Design review of the part shown in the three views and the two pictorial views. Dimensions are in mm from the part's minimum x, y and z. A direction names the side the tool comes from. Round coordinates to 2 decimals unless told otherwise and drop trailing zeros. Order: outer loops, then holes, each group sorted by start corner. A loop starts at its lowest first (then second) coordinate and runs counter-clockwise, first axis right, second up.
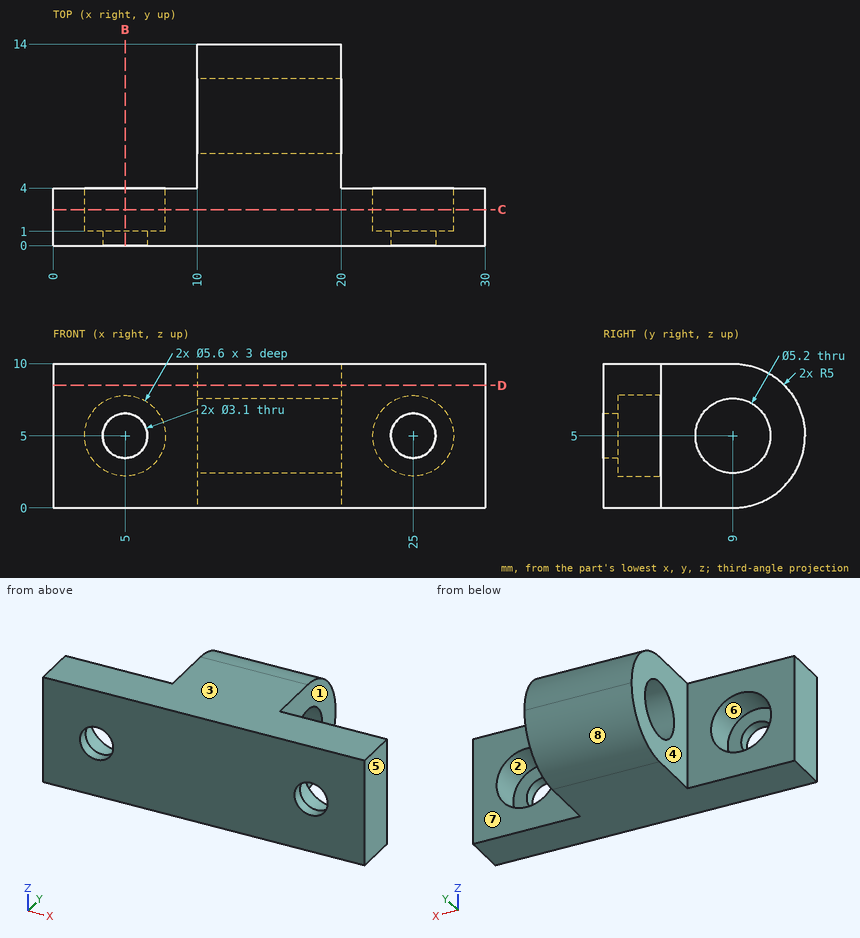
1) The part is to be moulded in two halves that separate along X. For the marked faces 1, 2 and 3, say which applies: released by +X, released by -X, zero draft, split by the parting line, or undercut.
Results:
face 1: released by +X
face 2: undercut
face 3: zero draft
2) To check wall thickness, follow line 1 along X through (y, z) = (2.75, 5); line 2 along Z through (x, y) = (5, 0.6); line 3 along Y through (x, z) = (14, 5). State the ranges of each line that lie inside material, in increasing order.
Results:
line 1: x = 0 to 2.2, 7.8 to 22.2, 27.8 to 30
line 2: z = 0 to 3.45, 6.55 to 10
line 3: y = 0 to 6.4, 11.6 to 14
3) Take a section at D-D on z = 8.5. Give the boundary of the cut face in (x, y), plus the area to 3 significant figures.
Results:
outline: (0, 0) - (30, 0) - (30, 4) - (20, 4) - (20, 12.57) - (10, 12.57) - (10, 4) - (0, 4) - close
area: 206 mm2
4) For the marked faces 4, 5, 6, 7 and 8, list the 3-axis set-ups (+Z, -Z, +X, -X, +Y, -Y) from which the entire face can be reached by the end or side of a thin tool; tool diameter is ignored.
Results:
face 4: +Z, -Z, -X, +Y
face 5: +Z, -Z, +X, +Y, -Y
face 6: +Y
face 7: +Z, -Z, +X, +Y
face 8: -Z, +X, -X, +Y
5) Take a section at C-C on y = 2.5. Give the boundary of the cut face in (x, z).
Results:
outline: (0, 0) - (30, 0) - (30, 10) - (0, 10) - close; hole circle Ø5.6 at (5, 5); hole circle Ø5.6 at (25, 5)
6) Take a section at B-B on x = 5. Give the boundary of the cut face in (y, z), plus the area to 3 significant figures.
Results:
outline: (0, 0) - (4, 0) - (4, 2.2) - (1, 2.2) - (1, 3.45) - (0, 3.45) - close; (0, 6.55) - (1, 6.55) - (1, 7.8) - (4, 7.8) - (4, 10) - (0, 10) - close
area: 20.1 mm2
7) Clearance check with flat-ended pins moving along their axes: P1, Ø1.7, axis at x = 26.5, z = 5.5, coming from the +Y side; P2, Ø5, axis at x = 4, z = 4, coming from the +Y side; P3, Ø6, axis at x = 22, y = 11.5, coming from the +Z side. State where each tip first meets the part, or that it passes through.
Results:
P1: stops at y = 1
P2: stops at y = 4
P3: stops at z = 9.99
